Could you check a few things on this drawing? It's one solid part, dimensions in mm from its lowest x, y, z. Coordinates: 2 decimals unless noted, no trailing zeros. Order: outer loops, then holes, each group sorted by start corner. A loop starts at its lowest first (then second) coordinate and runs counter-clockwise, first axis right, second up.
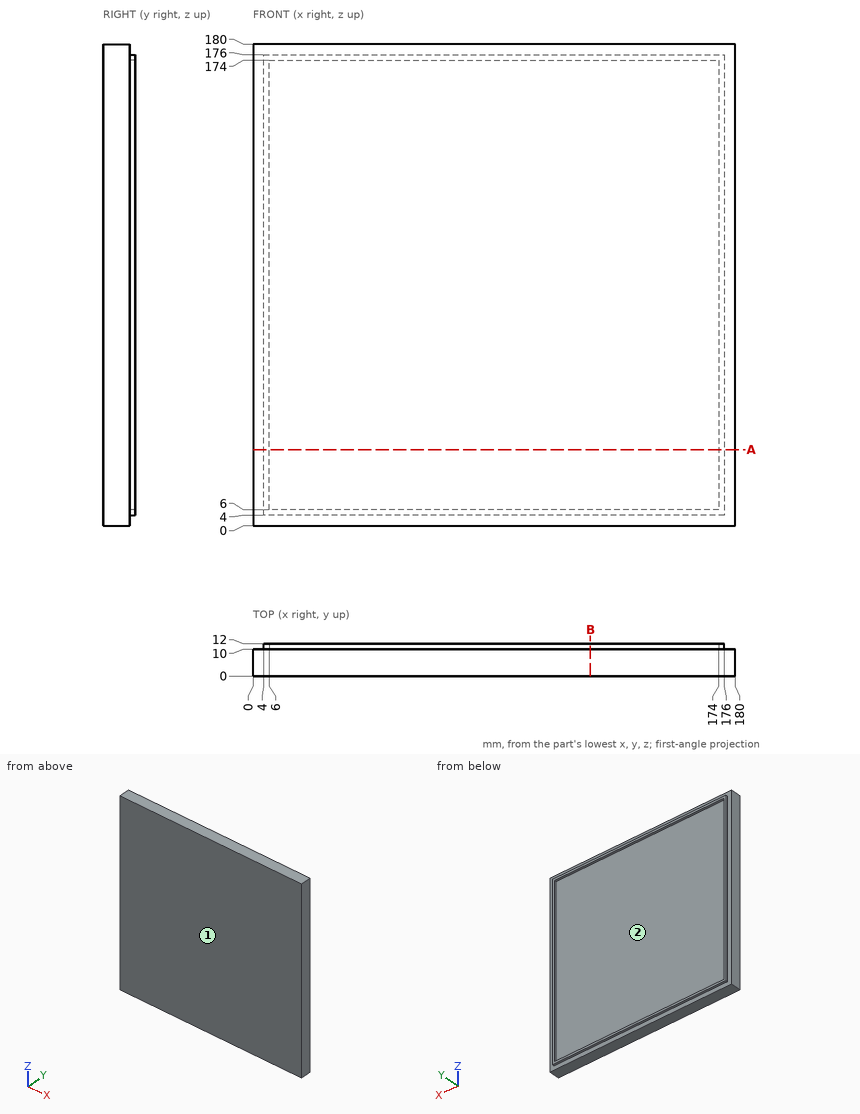
Item 1: For pin 1 Ø0.6 at (x, y) = (103.5, 11.5) entering from -Z; pin 2 Ø0.6 at (x, y) = (70, 11) entering from +Z; pin 3 Ø1.6 at (y, z) = (11, 123.5) entering from -X, each with a flat end and sliding along its axis, tell me the tip position at first contact or that it passes through.
Item 2: Thinking about a two-plate mould opening in Y: for the marked faces 1 and 2, which applies, +Y half, -Y half, draft (parallel to the pull), parting line (faces both ways), or undercut?
Item 3: Suppose I cut it at B-B (x = 126). List the corners of the cut face in (y, z) for me, and give its area (3 significant figures).
Item 4: I need wall thicknesses on line 1 (X direction, y = 11.25, z = 73); line 2 (Y direction, x = 90.5, z = 35). Which ranges of each line are inside material? Lowest first, please.
Item 5: Suppose I cut it at A-A (z = 28.5). List the corners of the cut face in (x, y) for me.
Geometry results:
1. pin 1: stops at z = 4
1. pin 2: stops at z = 176
1. pin 3: stops at x = 4
2. face 1: -Y half
2. face 2: +Y half
3. outline: (0, 0) - (10, 0) - (10, 4) - (12, 4) - (12, 6) - (10, 6) - (10, 174) - (12, 174) - (12, 176) - (10, 176) - (10, 180) - (0, 180) - close
3. area: 1,810 mm2
4. line 1: x = 4 to 6, 174 to 176
4. line 2: y = 0 to 10
5. outline: (0, 0) - (180, 0) - (180, 10) - (176, 10) - (176, 12) - (174, 12) - (174, 10) - (6, 10) - (6, 12) - (4, 12) - (4, 10) - (0, 10) - close
